For this review, take the finished solid that the model builds, in its own axes (mm). A direction names the side the tool comes from. Give positions to 0.01 mm unless a question says otherwise; leave off trailing zeros. Write each loop counter-clockwise with the first axis right and the second up, starting at its lowest first coordinate (ties: lowest second). Pieces come first, ordered by that corner, then holes.
Q1. Mouldability with a two-part tool opening along Y and no side actions: class faces 1 (the cylindrical face through (-3.905, 14.79, -0.867)), 2 (the flat face through (-4, 30, -3)), 3 (the cylindrical face through (-13.865, 4.57, 8.535)) as released by +Y, released by -Y, zero draft, split by the parting line, or undercut.
Q2. We need section B-B (x = 0). Write out the cut boundary in (y, z).
Q3. Machinability: for faces 4 (the flat face through (12, 6, 6)), 5 (the flat face through (-17, 15, 0)), which of the approach directions +Z, -Z, +X, -X, +Y, -Y give a long, thin tool a straight path to every point of the face, cutting with its end or side? Answer none if there is none.
Q4. We need section C-C (y = 27). Write out the cut boundary in (x, z), then the cut area to 3 significant figures.
Q5. We need section A-A (z = 0). Write out the cut boundary in (x, y), then the cut area to 3 significant figures.
Q6. For line 1 (Y direction, x = 12, z = 9.9); line 2 (X direction, y = 12.25, z = 0); line 3 (X direction, y = 17.75, z = -2.5), list the stretches that pass through material, from the lowest coordinate up.
Q7. We need section D-D (x = -12). Write out the cut boundary in (y, z).
Q8. Insertion check: P1, Ø1.4, axis at x = -12, y = 5.5, coming from the +Z side. The pin has a flat end and moves straight along its axis. Give the tip position at first contact, or say it passes through.
```python
from build123d import *

# Parameters (mm, degrees)
SKETCH1_W           = 34
SKETCH1_H           = 22
SKETCH1_R           = 4
BOSS_EXTRUDE1_DEPTH = 30
SKETCH3_R           = 2.35
CUT_EXTRUDE1_DEPTH  = 5


with BuildPart() as part:
    # Sketch1 → Boss-Extrude1 (new body)
    with BuildSketch(Plane(origin=(0, 0, 0), x_dir=(1, 0, 0), z_dir=(0, 1, 0))):
        Rectangle(SKETCH1_W, SKETCH1_H)
        with Locations(Location((0, 0, 0), (0, 0, 270))):
            Circle(SKETCH1_R, mode=Mode.SUBTRACT)
    extrude(amount=BOSS_EXTRUDE1_DEPTH)

    # Sketch3 → Cut-Extrude1 (cut)
    with BuildSketch(Plane.XY.offset(11)):
        with Locations((-12, 24)):
            Circle(SKETCH3_R)
        with Locations((-12, 6)):
            Circle(SKETCH3_R)
        with Locations(Location((12, 6, 0), (0, 0, 180))):
            Circle(SKETCH3_R)
        with Locations(Location((12, 24, 0), (0, 0, 180))):
            Circle(SKETCH3_R)
    extrude(amount=-CUT_EXTRUDE1_DEPTH, mode=Mode.SUBTRACT)


solid = part.part
```
Computed:
1. face 1: zero draft
1. face 2: released by +Y
1. face 3: undercut
2. outline: (0, -11) - (30, -11) - (30, -4) - (0, -4) - close; (0, 4) - (30, 4) - (30, 11) - (0, 11) - close
3. face 4: +Z
3. face 5: +Z, -Z, -X, +Y, -Y
4. outline: (-17, -11) - (17, -11) - (17, 11) - (-17, 11) - close; hole circle Ø8 at (0, 0)
4. area: 698 mm2
5. outline: (-17, 0) - (-4, 0) - (-4, 30) - (-17, 30) - close; (4, 0) - (17, 0) - (17, 30) - (4, 30) - close
5. area: 780 mm2
6. line 1: y = 0 to 3.65, 8.35 to 21.65, 26.35 to 30
6. line 2: x = -17 to -4, 4 to 17
6. line 3: x = -17 to -3.12, 3.12 to 17
7. outline: (0, -11) - (30, -11) - (30, 11) - (26.35, 11) - (26.35, 6) - (21.65, 6) - (21.65, 11) - (8.35, 11) - (8.35, 6) - (3.65, 6) - (3.65, 11) - (0, 11) - close
8. P1: stops at z = 6
